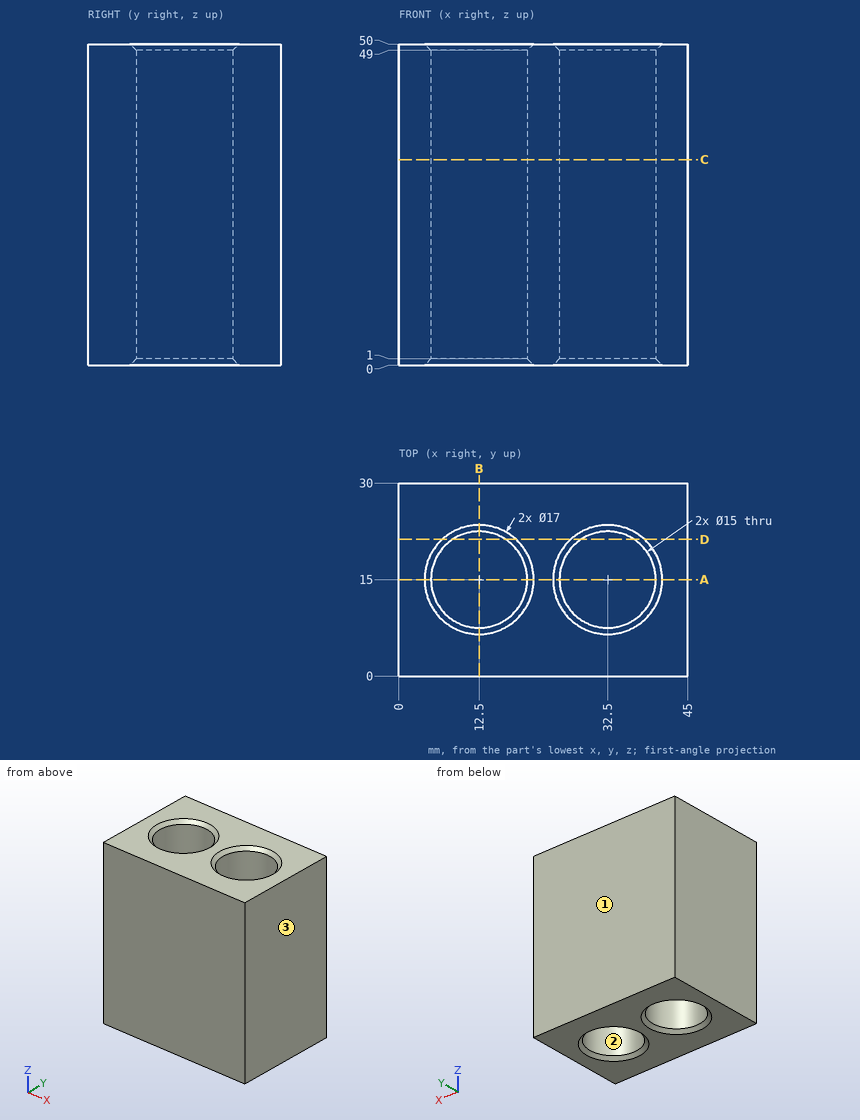
The figure shows three views and two pictorial views of one solid part (mm, origin at its lowest corner). Answer the questions. Give positions to 0.01 mm unless a question says otherwise; leave off trailing zeros. Write each loop counter-clockwise with the first axis right and the second up, starting at its lowest first coordinate (ties: lowest second). Pieces come first, ordered by that corner, then holes. Notation, with made-up numbers: (80, -20) - (93, -20) arc R13 cw to (93, 3) - close; hole circle Ø4 at (62, -15). An arc over 180 degrees is marked (long way). Use one line per item in the form item = value. Start each with the question number.
1) Consider line 1 along X through (y, z) = (11, 17); line 2 along Y through (x, z) = (32.5, 11.5); line 3 along X through (y, z) = (20.5, 19). Determine where each line is inside the solid, lowest interval first. Write a range as from..to.
2) Find section D-D on y = 21.25. Count the separate pieces of the cut face and the enclosed holes in it, plus the area to 3 significant figures.
3) Flat-ended cylindrical pins translate along their axes: pin 1 Ø5 at (y, z) = (5, 25) entering from -X; pin 2 Ø9 at (x, y) = (32.5, 15) entering from +Z. Find the tip coordinate at first contact, or state that the pin passes through.
4) Find section B-B on x = 12.5. Determine the outline of the cut face in (y, z), plus the area to 3 significant figures.
5) Find section C-C on z = 32. Determine the outline of the cut face in (x, y).
6) Find section A-A on y = 15. Determine the outline of the cut face in (x, z).
7) The mould has two halves that part along X. Classify the marked faces 1, 2 and 3: pulls with the +X half, pulls with the -X half, needs draft (parallel to the pull), parting line crosses it, or undercut.
Geometry results:
q1.line_1 = 0..6.16, 18.84..26.16, 38.84..45
q1.line_2 = 0..7.5, 22.5..30
q1.line_3 = 0..7.4, 17.6..27.4, 37.6..45
q2.separate_pieces = 3
q2.enclosed_holes = 0
q2.area = 1,410 mm2
q3.pin_1 = 0
q3.pin_2 = through
q4.outline = (0, 0) - (6.5, 0) - (7.5, 1) - (7.5, 49) - (6.5, 50) - (0, 50) - close; (22.5, 1) - (23.5, 0) - (30, 0) - (30, 50) - (23.5, 50) - (22.5, 49) - close
q4.area = 748 mm2
q5.outline = (0, 0) - (45, 0) - (45, 30) - (0, 30) - close; hole circle Ø15 at (12.5, 15); hole circle Ø15 at (32.5, 15)
q6.outline = (0, 0) - (4, 0) - (5, 1) - (5, 49) - (4, 50) - (0, 50) - close; (20, 1) - (21, 0) - (24, 0) - (25, 1) - (25, 49) - (24, 50) - (21, 50) - (20, 49) - close; (40, 1) - (41, 0) - (45, 0) - (45, 50) - (41, 50) - (40, 49) - close
q7.face_1 = needs draft
q7.face_2 = undercut
q7.face_3 = pulls with the +X half
